```python
from build123d import *

# Parameters (mm, degrees)
SKETCH_1_R      = 1.65
EXTRUDE_2_DEPTH = 10
FILLET_2_R      = 3


with BuildPart() as part:
    # ｽｹｯﾁ1 → ﾎﾞｽ - 押し出し2 (new body)
    with BuildSketch(Plane.XY):
        with BuildLine():
            ThreePointArc((13.495853088, -13.373927973), (-2.494791786, -18.835498771), (-16.512205084, -9.399312914))
            Line((-16.512205084, -9.399312914), (-27.997360851, 10.777188196))
            ThreePointArc((-27.997360851, 10.777188196), (-5.480838188, -29.495091333), (30, 0))
            ThreePointArc((30, 0), (29.95938456, 1.560537335), (29.837648215, 3.116849208))
            Line((29.837648215, 3.116849208), (13.495853088, -13.373927973))
        make_face()
        with Locations((-21.217622393, -12.25)):
            Circle(SKETCH_1_R, mode=Mode.SUBTRACT)
        with Locations((0, -24.5)):
            Circle(SKETCH_1_R, mode=Mode.SUBTRACT)
        with Locations((21.217622393, -12.25)):
            Circle(SKETCH_1_R, mode=Mode.SUBTRACT)
    extrude(amount=EXTRUDE_2_DEPTH)

    # ﾌｨﾚｯﾄ2
    fillet_2_edges = [part.edges().sort_by_distance(p)[0] for p in [
        (29.837648215, 3.116849208, 5),
        (-27.997360851, 10.777188196, 5),
    ]]
    fillet(fillet_2_edges, radius=FILLET_2_R)


solid = part.part
```
Can you work these out from the model? Positions are in its coordinate system, mm. A direction names the side the tool comes from. Round coordinates to 2 decimals unless told otherwise and drop trailing zeros. Loops run counter-clockwise (first coordinate to the right, second up) from the corner with the lowest first, then second, coordinate; pieces in that order, holes last.
Item 1: Suppose I cut it at C-C, the plane y = -12.25. Write out the boundary of the cut face in (x, z), then the cut area to 3 significant figures.
Item 2: If we mould it in two halves opening along Y, with no side actions, what happens to faces 3 (the flat face through (19.08, -7.74, 4.93)), 4 (the cylindrical face through (-22.53, -13.25, 4.93)), 5 (the flat face through (-1, -20, 10))? For each: +Y half, -Y half, draft (parallel to the pull), parting line (faces both ways), or undercut.
Item 3: Will these pins go through, and if not, where does the flat tip stop? pin 1 Ø5 at (x, z) = (13.5, 5) entering from +Y; pin 2 Ø3 at (x, z) = (-13, 1) entering from -Y; pin 3 Ø4 at (x, z) = (12.5, 8) entering from -Y.
Item 4: Suppose I cut it at B-B, the plane y = -24.5. Write out the boundary of the cut face in (x, z).
Item 5: Please list where these lines run through material, in increasing order: L1, parallel to Y at x = 0, z = 5.75; L2, parallel to X at y = -11.5, z = 1.5; L3, parallel to X at y = -6.5, z = 2.5.
Item 6: Suppose I cut it at D-D, the plane z = 8. State how many separate pieces and enclosed holes the cut face has, then the cut area to 3 significant figures.
Item 7: Suppose I cut it at A-A, the plane x = 0. Write out the boundary of the cut face in (y, z), then the cut area to 3 significant figures.
Item 8: Which directions (+Z, -Z, +X, -X, +Y, -Y) give clear straight access to the entire face, cutting with the end or side of a thin tool? Please do faces 1 (the flat face through (-1, -20, 0)), 2 (the flat face through (-20.33, -2.69, 4.93)).
Reported:
1. outline: (-27.38, 0) - (-22.87, 0) - (-22.87, 10) - (-27.38, 10) - close; (-19.57, 0) - (-14.52, 0) - (-14.52, 10) - (-19.57, 10) - close; (14.61, 0) - (19.57, 0) - (19.57, 10) - (14.61, 10) - close; (22.87, 0) - (27.38, 0) - (27.38, 10) - (22.87, 10) - close
1. area: 190 mm2
2. face 3: +Y half
2. face 4: undercut
2. face 5: draft
3. pin 1: stops at y = -10.85
3. pin 2: stops at y = -27.71
3. pin 3: stops at y = -28.1
4. outline: (-17.31, 0) - (-1.65, 0) - (-1.65, 10) - (-17.31, 10) - close; (1.65, 0) - (17.31, 0) - (17.31, 10) - (1.65, 10) - close
5. L1: y = -30 to -26.15, -22.85 to -19
5. L2: x = -27.71 to -22.69, -19.75 to -15.12, 15.35 to 19.75, 22.69 to 27.71
5. L3: x = -29.29 to -18.16, 20.31 to 29.29
6. separate pieces: 1
6. enclosed holes: 3
6. area: 800 mm2
7. outline: (-30, 0) - (-26.15, 0) - (-26.15, 10) - (-30, 10) - close; (-22.85, 0) - (-19, 0) - (-19, 10) - (-22.85, 10) - close
7. area: 77.0 mm2
8. face 1: -Z, +X, -X, +Y, -Y
8. face 2: +Z, -Z, +Y
